```python
from build123d import *

# Parameters (mm, degrees)
SKETCH1_R           = 12.7
SKETCH1_R_2         = 3.96875
BOSS_EXTRUDE1_DEPTH = 2.54
BOSS_EXTRUDE2_START = -88.9
SKETCH2_R           = 3.96875
BOSS_EXTRUDE2_DEPTH = 177.8


with BuildPart() as part:
    # Sketch1 → Boss-Extrude1 (new body)
    with BuildSketch(Plane(origin=(0, 0, 0), x_dir=(1, 0, 0), z_dir=(0, 1, 0))):
        with Locations(Location((0, 0, 0), (0, 0, 270))):
            Circle(SKETCH1_R)
        with Locations(Location((0, 0, 0), (0, 0, 270))):
            Circle(SKETCH1_R_2, mode=Mode.SUBTRACT)
    extrude(amount=BOSS_EXTRUDE1_DEPTH)

    # Sketch2 → Boss-Extrude2 (add)
    with BuildSketch(Plane(origin=(0, 2.54, 0), x_dir=(1, 0, 0), z_dir=(0, 1, 0)).offset(BOSS_EXTRUDE2_START)):
        with Locations(Location((0, 0, 0), (0, 0, 270))):
            Circle(SKETCH2_R)
    extrude(amount=BOSS_EXTRUDE2_DEPTH)

    # Sketch3 → Revolve1 (revolve)
    with BuildSketch(Plane(origin=(0, 0, 0), x_dir=(0, 0, -1), z_dir=(1, 0, 0))):
        Polygon((0, -86.36), (-3.96875, -86.36), (0, -91.517208385), align=None)
    revolve(axis=Axis((0, -87.920610372, 0), (0, 1, 0)))


solid = part.part
```
Verification items for the finished model (mm, model axes). A direction names the side the tool comes from. Round coordinates to 2 decimals unless told otherwise and drop trailing zeros. Loops run counter-clockwise (first coordinate to the right, second up) from the corner with the lowest first, then second, coordinate; pieces in that order, holes last. Notation, with made-up numbers: (-6, 61) -> (50, 61) arc R37 ccw to (50, 98) -> close; hole circle Ø4 at (62, -4). An arc over 180 degrees is marked (long way). Answer as a JSON object with one key per item and string values.
Q1. Scan lines: line 1 (X direction, y = -13, z = -0.25); line 2 (Y direction, x = -1, z = -5); line 3 (X direction, y = 13, z = -3). Record each from-to range of solid material in increasing order. Write a range as from..to.
Data:
{"line 1": "x = -3.96..3.96", "line 2": "y = 0..2.54", "line 3": "x = -2.6..2.6"}
Q2. Section check B-B (z = -10.5). Record the boundary of the cut face in (x, y), then the cut area to 3 significant figures.
Data:
{"outline": "(-7.14, 0) -> (7.14, 0) -> (7.14, 2.54) -> (-7.14, 2.54) -> close", "area": "36.3 mm2"}
Q3. Go/stop test with flat-tipped pins: P1, Ø4, axis at x = 1.5, z = 7, coming from the +Y side; P2, Ø10, axis at x = 6, y = -70, coming from the +Z side; P3, Ø7.5, axis at x = 5, z = -4.5, coming from the +Y side; P4, Ø2, axis at y = 7.5, z = 1.5, coming from the -X side. Record where each tip stops, or that it passes through.
Data:
{"P1": "stops at y = 2.54", "P2": "stops at z = 3.84", "P3": "stops at y = 91.44", "P4": "stops at x = -3.94"}
Q4. Access from +Z, -Z, +X, -X, +Y, -Y to the whole of each face (thin tool, end or side, straight path). Record for faces 1 (the cylindrical face through (-3.874, -43.785, -0.86)), 2 (the flat face through (3, 2.54, 3)), 3 (the cylindrical face through (-7.7, 1.3, -10.1)).
Data:
{"face 1": "-Y", "face 2": "+Y", "face 3": "+Y, -Y"}
Q5. Section check A-A (y = 46). Record the boundary of the cut face in (x, z).
Data:
{"outline": "circle Ø7.94 at (0, 0)"}
Q6. Section check C-C (x = -6.5). Record the boundary of the cut face in (y, z).
Data:
{"outline": "(0, -10.91) -> (2.54, -10.91) -> (2.54, 10.91) -> (0, 10.91) -> close"}
